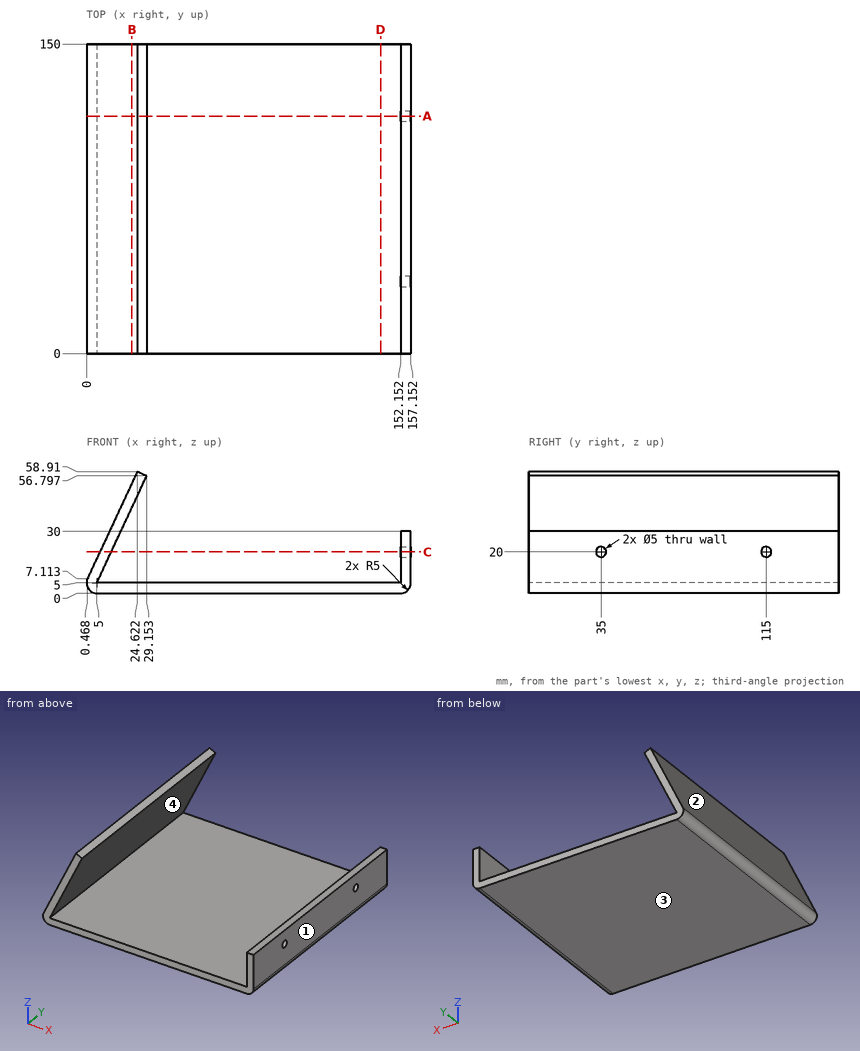
Could you check a few things on this drawing? It's one solid part, dimensions in mm from its lowest x, y, z. Round coordinates to 2 decimals unless told otherwise and drop trailing zeros. Loops run counter-clockwise (first coordinate to the right, second up) from the corner with the lowest first, then second, coordinate; pieces in that order, holes last. Notation, with made-up numbers: (-14, 67.25) -> (25, 67.25) arc R24 cw to (25, 80.25) -> close; hole circle Ø10 at (12, -31.75). An arc over 180 degrees is marked (long way). One line per item, written item: value. Start each with the question number.
1. If we section it at A-A, the plane y = 115: Write out the boundary of the cut face in (x, z).
2. If we mould it in two halves opening along X, with no side actions, what happens to the marked faces 1, 2, 3 and 4? For each: pulls with the +X half, pulls with the -X half, needs draft (parallel to the pull), parting line crosses it, or undercut.
3. If I drill on probe 1 along Z at (x, y) = (99, 8.5); probe 2 along X at (y, z) = (22, 19); probe 3 along X at (y, z) = (138, 27), over which ranges is the centre line in solid material (lowest first)?
4. If we section it at C-C, the plane z = 20: Write out the boundary of the cut face in (x, y) (1 decimal), then the cut area to 3 significant figures.
5. If we section it at B-B, the plane x = 22: Write out the boundary of the cut face in (y, z).
6. For pin 1 (4 mm diameter, centred on x = 20.5, y = 26.5, fed in from +Z); pin 2 (6 mm diameter, centred on y = 115, z = 20, fed in from -X); pin 3 (1.5 mm diameter, centred on x = 153.5, y = 80.5, fed in from +Z), each with a flat end and sliding along its axis, tell me the tip position at first contact or that it passes through.
7. If we section it at D-D, the plane x = 142.5: Write out the boundary of the cut face in (y, z).
Calculated:
1. outline: (0.47, 7.11) arc R5 ccw to (5, 0) -> (152.15, 0) arc R5 ccw to (157.15, 5) -> (157.15, 17.5) -> (152.15, 17.5) -> (152.15, 5) -> (5, 5) -> (29.15, 56.8) -> (24.62, 58.91) -> close; (152.15, 22.5) -> (157.15, 22.5) -> (157.15, 30) -> (152.15, 30) -> close
2. face 1: pulls with the +X half
2. face 2: pulls with the -X half
2. face 3: needs draft
2. face 4: undercut
3. probe 1: z = 0 to 5
3. probe 2: x = 6.01 to 11.53, 152.15 to 157.15
3. probe 3: x = 9.74 to 15.26, 152.15 to 157.15
4. outline: (6.5, 0) -> (12, 0) -> (12, 150) -> (6.5, 150) -> close; (152.2, 0) -> (157.2, 0) -> (157.2, 32.5) -> (152.2, 32.5) -> close; (152.2, 37.5) -> (157.2, 37.5) -> (157.2, 112.5) -> (152.2, 112.5) -> close; (152.2, 117.5) -> (157.2, 117.5) -> (157.2, 150) -> (152.2, 150) -> close
4. area: 1,530 mm²
5. outline: (0, 0) -> (150, 0) -> (150, 5) -> (0, 5) -> close; (0, 41.46) -> (150, 41.46) -> (150, 53.29) -> (0, 53.29) -> close
6. pin 1: stops at z = 54.36
6. pin 2: stops at x = 5.08
6. pin 3: stops at z = 30
7. outline: (0, 0) -> (150, 0) -> (150, 5) -> (0, 5) -> close
